Source: CAD feature listing. Evaluate the final solid. Frame: model axes, mm. Face numbers are marked on the shaded views. A direction names the side the tool comes from. Give positions to 0.01 mm unless a question says otherwise; leave off trailing zeros. Loops run counter-clockwise (first coordinate to the right, second up) from the corner with the lowest first, then second, coordinate; pieces in that order, holes last. Notation, with made-up numbers: (0, 61) - (24, 61) arc R21 cw to (24, 79) - close; hole circle Ø3 at (-4.75, -17.5). An arc over 180 degrees is marked (long way). Put each result on its own line as item: value.
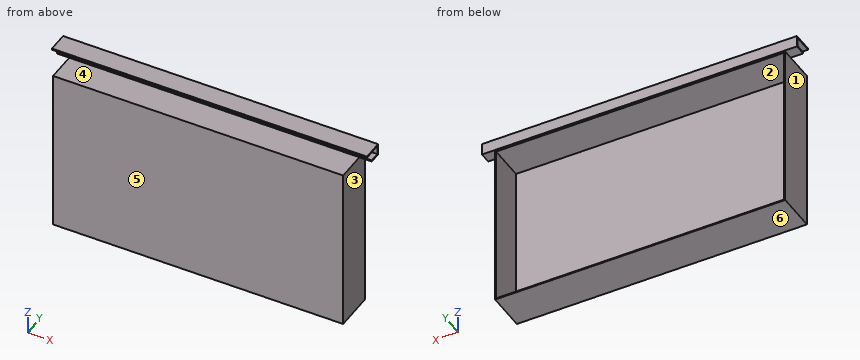
```python
from build123d import *

# Parameters (mm, degrees)
SKETCH1_W         = 222.25
SKETCH1_H         = 127
SKETCH1_W_2       = 220.7514
SKETCH1_H_2       = 125.5014
BASE_DEPTH        = 2.54
SKETCH1_3_W       = 222.25
SKETCH1_3_H       = 127
SKETCH1_3_W_2     = 220.7514
SKETCH1_3_H_2     = 125.5014
WALLS_DEPTH       = 30.1625
HANDLE_DEPTH      = 120.65
HANDLE_DEPTH_BACK = 120.65


with BuildPart() as part:
    # Sketch1 → Base (new body)
    # profile 1 of 2: a face of its own
    with BuildSketch(Plane(origin=(0, 0, 0), x_dir=(1, 0, 0), z_dir=(0, 1, 0))):
        with Locations((0, 63.5)):
            Rectangle(SKETCH1_W, SKETCH1_H)
    # profile 2 of 2: a face of its own
    with BuildSketch(Plane(origin=(0, 0, 0), x_dir=(1, 0, 0), z_dir=(0, 1, 0))):
        with Locations((0, 63.5)):
            Rectangle(SKETCH1_W, SKETCH1_H)
        with Locations((0, 63.5)):
            Rectangle(SKETCH1_W_2, SKETCH1_H_2, mode=Mode.SUBTRACT)
    extrude(amount=BASE_DEPTH)

    # Sketch1_3 → Walls (add)
    with BuildSketch(Plane(origin=(0, 0, 0), x_dir=(1, 0, 0), z_dir=(0, 1, 0))):
        with Locations((0, 63.5)):
            Rectangle(SKETCH1_3_W, SKETCH1_3_H)
        with Locations((0, 63.5)):
            Rectangle(SKETCH1_3_W_2, SKETCH1_3_H_2, mode=Mode.SUBTRACT)
    extrude(amount=WALLS_DEPTH)

    # Sketch2 → Handle (add, two sides: drawn at the far end of the back side and taken through both)
    with BuildSketch(Plane(origin=(0, 0, 0), x_dir=(0, 0, -1), z_dir=(1, 0, 0)).offset(-HANDLE_DEPTH_BACK)):
        Polygon((0, 22.475414602), (0, 31.1785), (-8.89, 31.1785), (-8.89, 15.6845), (-7.874, 15.6845), (-7.874, 30.1625), (-1.016, 30.1625), (-1.016, 22.475414602), align=None)
    extrude(amount=HANDLE_DEPTH + HANDLE_DEPTH_BACK)


solid = part.part
```
1) Pin query (flat end, axial travel): P1, Ø10, axis at x = 28.5, z = -107, coming from the -Y side; P2, Ø0.5, axis at x = 21.5, z = 0.5, coming from the -Y side; P3, Ø9, axis at y = 8.5, z = -41.5, coming from the -X side (3 decimals); P4, Ø10, axis at y = 22.5, z = -107.5, coming from the +X side (3 decimals). Return the tip coordinate at first contact, or that it passes through.
Check result:
P1: y = 0
P2: y = 22.48
P3: x = -111.125
P4: x = 111.125
2) Section query A-A, the plane y = 27. Output: boundary loops of the cut face in (x, z) (3 decimals), plus the area to 3 significant figures.
Check result:
outline: (-120.65, 0) - (-111.125, 0) - (-111.125, -127) - (111.125, -127) - (111.125, 0) - (120.65, 0) - (120.65, 1.016) - (-120.65, 1.016) - close; (-120.65, 7.874) - (120.65, 7.874) - (120.65, 8.89) - (-120.65, 8.89) - close; hole (-110.376, -126.251) - (110.376, -126.251) - (110.376, -0.749) - (-110.376, -0.749) - close
area: 1,010 mm²
3) Section query B-B, the plane x = 15.5. Output: boundary loops of the cut face in (y, z), plus the area to 3 significant figures.
Check result:
outline: (0, -127) - (30.16, -127) - (30.16, -126.25) - (2.54, -126.25) - (2.54, -0.75) - (30.16, -0.75) - (30.16, 0) - (31.18, 0) - (31.18, 8.89) - (15.68, 8.89) - (15.68, 7.87) - (30.16, 7.87) - (30.16, 1.02) - (22.48, 1.02) - (22.48, 0) - (0, 0) - close
area: 396 mm²
4) Material intervals for line 1 along Z through (x, y) = (44, 17); line 2 along Z through (x, y) = (-49, 24); line 3 along X through (y, z) = (11, -18.5) (3 decimals), sorted ascending. Write a range as [from, to].
Check result:
line 1: [-127, -126.25], [-0.75, 0], [7.87, 8.89]
line 2: [-127, -126.25], [-0.75, 1.02], [7.87, 8.89]
line 3: [-111.125, -110.376], [110.376, 111.125]
5) Section query D-D, the plane y = 9. Output: boundary loops of the cut face in (x, z) (3 decimals), plus the area to 3 significant figures.
Check result:
outline: (-111.125, -127) - (111.125, -127) - (111.125, 0) - (-111.125, 0) - close; hole (-110.376, -126.251) - (110.376, -126.251) - (110.376, -0.749) - (-110.376, -0.749) - close
area: 521 mm²
6) Section query C-C, the plane z = -47.5. Output: boundary loops of the cut face in (x, y) (1 decimal).
Check result:
outline: (-111.1, 0) - (111.1, 0) - (111.1, 30.2) - (110.4, 30.2) - (110.4, 2.5) - (-110.4, 2.5) - (-110.4, 30.2) - (-111.1, 30.2) - close
7) Mould query, pull axis Z, two halves, no side actions, for the marked faces 4, 5 and 6. Classes: pulls with the +Z half, pulls with the -Z half, needs draft (parallel to the pull), parting line crosses it, or undercut.
Check result:
face 4: undercut
face 5: needs draft
face 6: pulls with the -Z half
8) Access query for the marked faces 1, 2 and 3. Directions: +Z, -Z, +X, -X, +Y, -Y. A direction counts if a zero-diameter tool reaches every point of the face in a straight line with its end or side. Return the directions, or none.
Check result:
face 1: -Z, -X, +Y, -Y
face 2: +Y
face 3: -Z, +X, +Y, -Y
